Check sheet for the modelled part. Datum: model origin and axes. Units: mm. A direction names the side the tool comes from. Give positions to 0.01 mm unless a question says otherwise; leave off trailing zeros. Order: outer loops, then holes, each group sorted by start corner. A loop starts at its lowest first (then second) coordinate and runs counter-clockwise, first axis right, second up.
from build123d import *

# Parameters (mm, degrees)
EXTRUDE_1_DEPTH     = 10
SKETCH_2_R          = 1.6
CUT_EXTRUDE_1_DEPTH = 20.798989873
SKETCH_4_W          = 10
SKETCH_4_H          = 5
CUT_EXTRUDE_2_DEPTH = 20
EXTRUDE_2_DEPTH     = 8
CUT_EXTRUDE_START   = -1
CUT_EXTRUDE_3_DEPTH = 1


# Read off the part's stored shape, not the designer's step: 除料-伸長3
with BuildPart() as part:
    # 草圖1 → 填料-伸長1 (new body)
    with BuildSketch(Plane(origin=(0, 0, 0), x_dir=(0, 0, -1), z_dir=(1, 0, 0))):
        Polygon((0, 0), (6, 0), (6, 1), (1, 1), (1, 16), (0, 16), align=None)
    extrude(amount=EXTRUDE_1_DEPTH)

    # 草圖2 → 除料-伸長1 (cut, through all)
    with BuildSketch(Plane.XY):
        with Locations((5, 11)):
            Circle(SKETCH_2_R)
        with Locations((5, 5)):
            Circle(SKETCH_2_R)
    extrude(amount=-CUT_EXTRUDE_1_DEPTH, mode=Mode.SUBTRACT)

    # 草圖4 → 除料-伸長2 (cut, through all)
    with BuildSketch(Plane(origin=(0, 1, 0), x_dir=(1, 0, 0), z_dir=(0, 1, 0))):
        with Locations((5, 3.5)):
            Rectangle(SKETCH_4_W, SKETCH_4_H)
    extrude(amount=-CUT_EXTRUDE_2_DEPTH, mode=Mode.SUBTRACT)

    # 草圖5 → 填料-伸長2 (add)
    with BuildSketch(Plane(origin=(0, 0, -1), x_dir=(-1, 0, 0), z_dir=(0, 0, -1))):
        with BuildLine():
            Line((2.524443153, 1.326762343), (2.18242301, 2.266454963))
            ThreePointArc((2.18242301, 2.266454963), (-5, 1), (-12.18242301, 2.266454963))
            Line((-12.18242301, 2.266454963), (-12.524443153, 1.326762343))
            ThreePointArc((-12.524443153, 1.326762343), (-5, 0), (2.524443153, 1.326762343))
        make_face()
    extrude(amount=EXTRUDE_2_DEPTH)

    # 除料-伸長3 outline → 除料-伸長3 (cut)
    with BuildSketch(Plane(origin=(0, 0, -1), x_dir=(-1, 0, 0), z_dir=(0, 0, -1)).offset(CUT_EXTRUDE_START)):
        with BuildLine():
            Line((0, 0), (0, 0.575714714))
            ThreePointArc((0, 0.575714714), (-2.483482164, 0.144402594), (-4.999999936, 0))
            Line((-4.999999936, 0), (0, 0))
        make_face()
        with BuildLine():
            Line((-10, 0), (-4.999999936, 0))
            ThreePointArc((-4.999999936, 0), (-7.516517772, 0.144402587), (-10, 0.575714714))
            Line((-10, 0.575714714), (-10, 0))
        make_face()
    extrude(amount=CUT_EXTRUDE_3_DEPTH, mode=Mode.SUBTRACT)


solid = part.part
1) Set-up check for faces 1 (the face through (5, 1, -5)), 2 (the face through (-1, 1, -1)), 3 (the face through (11, 1, -1)), 4 (the face through (5, 8, 0)): record each of +Z, -Z, +X, -X, +Y, -Y from which the full face is reachable in a straight line by a thin tool's end or side.
Recorded:
face 1: -Z, +Y
face 2: +Z, -X, +Y, -Y
face 3: +Z, +X, +Y, -Y
face 4: +Z, +X, -X, +Y, -Y
2) Material ranges on L1, parallel to Y at x = 5, z = -0.7; L2, parallel to Y at x = 4.75, z = -2.5; L3, parallel to Z at x = 4.75, y = 3, recorded low to high.
Recorded:
L1: y = 0 to 3.4, 6.6 to 9.4, 12.6 to 16
L2: y = 0 to 1
L3: z = -1 to 0
3) Draft check along Y on faces 5 (the face through (4.9, 16, -0.5)), 6 (the face through (4.65, 3.44, -0.49)), 7 (the face through (3.82, 12.08, -0.49)), 8 (the face through (5.1, 0.6, -9)). Enter one of: +Y half, -Y half, draft (parallel to the pull), parting line (faces both ways), or undercut.
Recorded:
face 5: +Y half
face 6: undercut
face 7: undercut
face 8: draft
4) Section check B-B, the plane y = 10. Record the cut outline in (x, z).
Recorded:
outline: (0, -1) - (3.75, -1) - (3.75, 0) - (0, 0) - close; (6.25, -1) - (10, -1) - (10, 0) - (6.25, 0) - close
5) Depth check by flat-ended pin: pin 1 Ø1.4 at (x, y) = (-1, 1.5) entering from +Z; pin 2 Ø2 at (y, z) = (7.5, -1.5) entering from +X; pin 3 Ø1.1 at (y, z) = (5.5, -0.5) entering from -X; pin 4 Ø4 at (x, y) = (5, 11) entering from +Z. Enter the tip coordinate at first touch or a pass-through.
Recorded:
pin 1: stops at z = -1
pin 2: stops at x = 10
pin 3: stops at x = 0
pin 4: stops at z = 0
6) Section check D-D, the plane y = 7.75. Record the cut outline in (x, z).
Recorded:
outline: (0, -1) - (10, -1) - (10, 0) - (0, 0) - close
7) Section check A-A, the plane y = 5. Record the cut outline in (x, z).
Recorded:
outline: (0, -1) - (3.4, -1) - (3.4, 0) - (0, 0) - close; (6.6, -1) - (10, -1) - (10, 0) - (6.6, 0) - close
8) Section check C-C, the plane z = -3. Record the cut outline in (x, y).
Recorded:
outline: (-2.52, 1.33) arc R22 ccw to (12.52, 1.33) - (12.18, 2.27) arc R21 cw to (-2.18, 2.27) - close
